from build123d import *

# Parameters (mm, degrees)
BASE_EXTRUDE_DEPTH  = 6
SKETCH2_R           = 9
BOSS_EXTRUDE1_DEPTH = 11
SKETCH3_R           = 9
BOSS_EXTRUDE2_DEPTH = 4
BOSS_EXTRUDE3_DEPTH = 6
SKETCH5_R           = 9
BOSS_EXTRUDE4_DEPTH = 26


with BuildPart() as part:
    # Sketch1 → Base-Extrude (new body)
    with BuildSketch(Plane.XY):
        Polygon((13.856406461, 0), (6.92820323, 12), (-6.92820323, 12), (-13.856406461, 0), (-6.92820323, -12), (6.92820323, -12), align=None)
    extrude(amount=BASE_EXTRUDE_DEPTH)

    # Sketch2 → Boss-Extrude1 (add)
    with BuildSketch(Plane.XY.offset(6)):
        Circle(SKETCH2_R)
    extrude(amount=BOSS_EXTRUDE1_DEPTH)

    # Sketch3 → Boss-Extrude2 (add)
    with BuildSketch(Plane(origin=(0, 0, 0), x_dir=(-1, 0, 0), z_dir=(0, 0, -1))):
        Circle(SKETCH3_R)
    extrude(amount=BOSS_EXTRUDE2_DEPTH)

    # Sketch4 → Boss-Extrude3 (add)
    with BuildSketch(Plane(origin=(0, 0, -4), x_dir=(-1, 0, 0), z_dir=(0, 0, -1))):
        Polygon((13.856406461, 0), (6.92820323, 12), (-6.92820323, 12), (-13.856406461, 0), (-6.92820323, -12), (6.92820323, -12), align=None)
    extrude(amount=BOSS_EXTRUDE3_DEPTH)

    # Sketch5 → Boss-Extrude4 (add)
    with BuildSketch(Plane(origin=(0, 0, -10), x_dir=(-1, 0, 0), z_dir=(0, 0, -1))):
        Circle(SKETCH5_R)
    extrude(amount=BOSS_EXTRUDE4_DEPTH)

    # Sketch8 → Cut-Revolve1 (revolve, cut)
    with BuildSketch(Plane(origin=(0, 0, 0), x_dir=(0, 0, -1), z_dir=(1, 0, 0))):
        Polygon((36, 0), (36, 7.147805433), (30.6, 6), (28.6, 6), (28.6, 5), (-9.6, 5), (-9.6, 6), (-11.6, 6), (-17, 7.147805433), (-17, 0), align=None)
    revolve(axis=Axis((0, 0, 19), (0, 0, -1)), mode=Mode.SUBTRACT)


solid = part.part
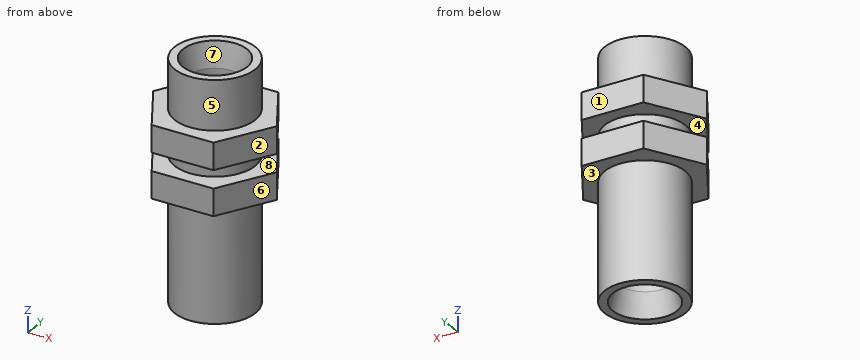
Design review of the part built by this model. Coordinates are the model's own, in mm. Face numbers are marked on the shaded views. A direction names the side the tool comes from. Coordinates: 2 decimals unless noted, no trailing zeros. Loops run counter-clockwise (first coordinate to the right, second up) from the corner with the lowest first, then second, coordinate; pieces in that order, holes last. Notation, with made-up numbers: M 64.25,-19 L 97.25,-19 A18 cw 97.25,6 Z; hole C 40,29 d1. An arc over 180 degrees is marked long. Answer as CSV lines item,"result".
Item 1: Add section D-D on z = -21.5. State the section outline as (x, y) points.
Answer list:
outline,"C 0,0 d18; hole C 0,0 d10"
Item 2: Machinability: for the marked faces 1, 2, 3, 4 and 5, which of the approach directions +Z, -Z, +X, -X, +Y, -Y give a long, thin tool a straight path to every point of the face, cutting with its end or side? Answer none if there is none.
Answer list:
face 1,"+Z, -Z, +X, -X, +Y"
face 2,"+Z, -Z, +X, -Y"
face 3,"-Z"
face 4,"none"
face 5,"+Z"
Item 3: Add section C-C on x = -8. State the section outline as (y, z) points.
Answer list:
outline,"M -10.14,-10 L -4.12,-10 L -4.12,-36 L 4.12,-36 L 4.12,-10 L 10.14,-10 L 10.14,-4 L 4.12,-4 L 4.12,0 L 10.14,0 L 10.14,6 L 4.12,6 L 4.12,17 L -4.12,17 L -4.12,6 L -10.14,6 L -10.14,0 L -4.12,0 L -4.12,-4 L -10.14,-4 Z"
Item 4: The part is to be moulded in two halves that separate along Y. For the marked faces 6, 7 and 8, say which applies: pulls with the +Y half, pulls with the -Y half, needs draft (parallel to the pull), parting line crosses it, or undercut.
Answer list:
face 6,"pulls with the -Y half"
face 7,"undercut"
face 8,"needs draft"
Item 5: For probe 1 along Z at (x, y) = (3, 11.25); probe 2 along X at (y, z) = (0, -9); probe 3 along X at (y, z) = (-0.25, -11.5), list the stretches that pass through material, from the lowest coordinate up.
Answer list:
probe 1,"-10 to -4, 0 to 6"
probe 2,"-13.86 to -5, 5 to 13.86"
probe 3,"-9 to -4.99, 4.99 to 9"
Item 6: Add section A-A on z = 3. State the section outline as (x, y) points.
Answer list:
outline,"M -13.86,0 L -6.93,-12 L 6.93,-12 L 13.86,0 L 6.93,12 L -6.93,12 Z; hole C 0,0 d10"
Item 7: For P1, Ø6, axis at x = 2.5, y = -0.5, coming from the +Z side; P2, Ø4, axis at x = 2.5, z = -18.5, coming from the -Y side; P3, Ø1.5, axis at x = -9, y = 4.5, coming from the -Z side, all flat-tipped, find the tip position at first contact; note any pin that passes through.
Answer list:
P1,"z = 9.6"
P2,"y = -8.99"
P3,"z = -10"
Item 8: Add section B-B on x = 12.25. State the section outline as (y, z) points, plus the area to 3 significant figures.
Answer list:
outline,"M -2.78,-10 L 2.78,-10 L 2.78,-4 L -2.78,-4 Z; M -2.78,0 L 2.78,0 L 2.78,6 L -2.78,6 Z"
area,"66.8 mm²"
